Can you work these out from the model? Positions are in its coordinate system, mm. A direction names the side the tool comes from. Coordinates: 2 decimals unless noted, no trailing zeros. Loops run counter-clockwise (first coordinate to the right, second up) from the corner with the lowest first, then second, coordinate; pieces in that order, holes last. Notation, with made-up numbers: (34.5, 84.25) -> (87.5, 84.25) arc R8 cw to (87.5, 97.25) -> close; hole circle Ø7 at (14, 50). An arc over 180 degrees is marked (long way). Use one line per item in the form item = value. Start each with the question number.
(1) Imagine slicing it at B-B (y = 9). List the corners of the cut face in (x, z) for me.
(2) Thinking about a two-plate mould opening in X: for faces 1 (the flat face through (0, 33, -25)), 2 (the cylindrical face through (-23.14, 18.25, -25.85)), 3 (the flat face through (-5, 18, 26.75)), which applies, released by +X, released by -X, zero draft, split by the parting line, or undercut?
(3) Imagine slicing it at D-D (y = 18.5). List the corners of the cut face in (x, z) for me.
(4) On a 3-axis mill with a long thin cutter (end or side, diameter ignored), from which of +Z, -Z, +X, -X, +Y, -Y can I reach the whole of each face in a straight line? I mean faces 4 (the flat face through (-5, 18, 23.75)), 5 (the flat face through (-24, 18, 0)), 6 (the flat face through (-1, 20, 25)), 7 (the cylindrical face through (22.48, 7.19, -0.91)), 8 (the flat face through (-9, 31, -25)). Say none if no direction works.
(5) Imagine slicing it at C-C (z = -20). List the corners of the cut face in (x, y) for me, plus the area to 3 significant figures.
(6) Imagine slicing it at A-A (z = -2.75). List the corners of the cut face in (x, y) for me.
(7) I need wall thicknesses on line 1 (Z direction, x = -13, y = 27); line 2 (X direction, y = 5, z = 10); line 3 (Y direction, x = 22.3, z = -2.75). Which ranges of each line are inside material? Lowest first, please. Write a range as [from, to].
(8) I'm going to push flat-ended pins straight in: pin 1 (1.5 mm diameter, centred on x = 12.5, y = 26, fed in from +Z); pin 2 (0.9 mm diameter, centred on y = 24, z = 25, fed in from -X); pin 3 (4.5 mm diameter, centred on y = 5.5, z = -2.75, fed in from +X). Where does each tip first touch, or does it pass through?
```python
from build123d import *

# Parameters (mm, degrees)
SKETCH1_W           = 48
SKETCH1_H           = 53.5
SKETCH1_W_2         = 42
SKETCH1_H_2         = 47.5
BOSS_EXTRUDE1_DEPTH = 36
SKETCH2_R           = 2.5
CUT_EXTRUDE1_DEPTH  = 9
SKETCH4_W           = 14.5
SKETCH4_H           = 15
CUT_EXTRUDE2_DEPTH  = 15
SKETCH6_W           = 18
SKETCH6_H           = 4
CUT_EXTRUDE3_DEPTH  = 15
FILLET1_R           = 3


with BuildPart() as part:
    # Sketch1 → Boss-Extrude1 (new body)
    with BuildSketch(Plane(origin=(0, 0, 0), x_dir=(1, 0, 0), z_dir=(0, 1, 0))):
        Rectangle(SKETCH1_W, SKETCH1_H)
        Rectangle(SKETCH1_W_2, SKETCH1_H_2, mode=Mode.SUBTRACT)
    extrude(amount=BOSS_EXTRUDE1_DEPTH)

    # Sketch2 → Cut-Extrude1 (cut)
    with BuildSketch(Plane(origin=(21, 0, 0), x_dir=(0, 0, -1), z_dir=(1, 0, 0))):
        with Locations((2.75, 5.5)):
            Circle(SKETCH2_R)
    extrude(amount=CUT_EXTRUDE1_DEPTH, mode=Mode.SUBTRACT)

    # Sketch4 → Cut-Extrude2 (cut)
    with BuildSketch(Plane.XY.offset(23.75)):
        with Locations((6.25, 20.5)):
            Rectangle(SKETCH4_W, SKETCH4_H)
    extrude(amount=CUT_EXTRUDE2_DEPTH, mode=Mode.SUBTRACT)

    # Sketch6 → Cut-Extrude3 (cut)
    with BuildSketch(Plane.XY.offset(-23.75)):
        with Locations((-9, 33)):
            Rectangle(SKETCH6_W, SKETCH6_H)
    extrude(amount=-CUT_EXTRUDE3_DEPTH, mode=Mode.SUBTRACT)

    # Fillet1
    fillet1_edges = [part.edges().sort_by_distance(p)[0] for p in [
        (24, 18, 26.75),
        (-24, 18, 26.75),
        (-24, 18, -26.75),
        (24, 18, -26.75),
    ]]
    fillet(fillet1_edges, radius=FILLET1_R)


solid = part.part
```
Worked out:
q1.outline = (-24, -23.75) arc R3 ccw to (-21, -26.75) -> (21, -26.75) arc R3 ccw to (24, -23.75) -> (24, 23.75) arc R3 ccw to (21, 26.75) -> (-21, 26.75) arc R3 ccw to (-24, 23.75) -> close; hole (-21, -23.75) -> (21, -23.75) -> (21, 23.75) -> (-21, 23.75) -> close
q2.face_1 = undercut
q2.face_2 = released by -X
q2.face_3 = zero draft
q3.outline = (-24, -23.75) arc R3 ccw to (-21, -26.75) -> (21, -26.75) arc R3 ccw to (24, -23.75) -> (24, 23.75) arc R3 ccw to (21, 26.75) -> (13.5, 26.75) -> (13.5, 23.75) -> (21, 23.75) -> (21, -23.75) -> (-21, -23.75) -> (-21, 23.75) -> (-1, 23.75) -> (-1, 26.75) -> (-21, 26.75) arc R3 ccw to (-24, 23.75) -> close
q4.face_4 = +Y, -Y
q4.face_5 = +Z, -Z, -X, +Y, -Y
q4.face_6 = +Z
q4.face_7 = +X
q4.face_8 = -Z
q5.outline = (-24, 0) -> (-21, 0) -> (-21, 36) -> (-24, 36) -> close; (21, 0) -> (24, 0) -> (24, 36) -> (21, 36) -> close
q5.area = 216 mm2
q6.outline = (-24, 0) -> (-21, 0) -> (-21, 36) -> (-24, 36) -> close; (21, 0) -> (24, 0) -> (24, 3) -> (21, 3) -> close; (21, 8) -> (24, 8) -> (24, 36) -> (21, 36) -> close
q7.line_1 = [-26.75, -23.75], [23.75, 26.75]
q7.line_2 = [-24, -21], [21, 24]
q7.line_3 = [0, 3], [8, 36]
q8.pin_1 = -23.75
q8.pin_2 = -23.89
q8.pin_3 = -21
